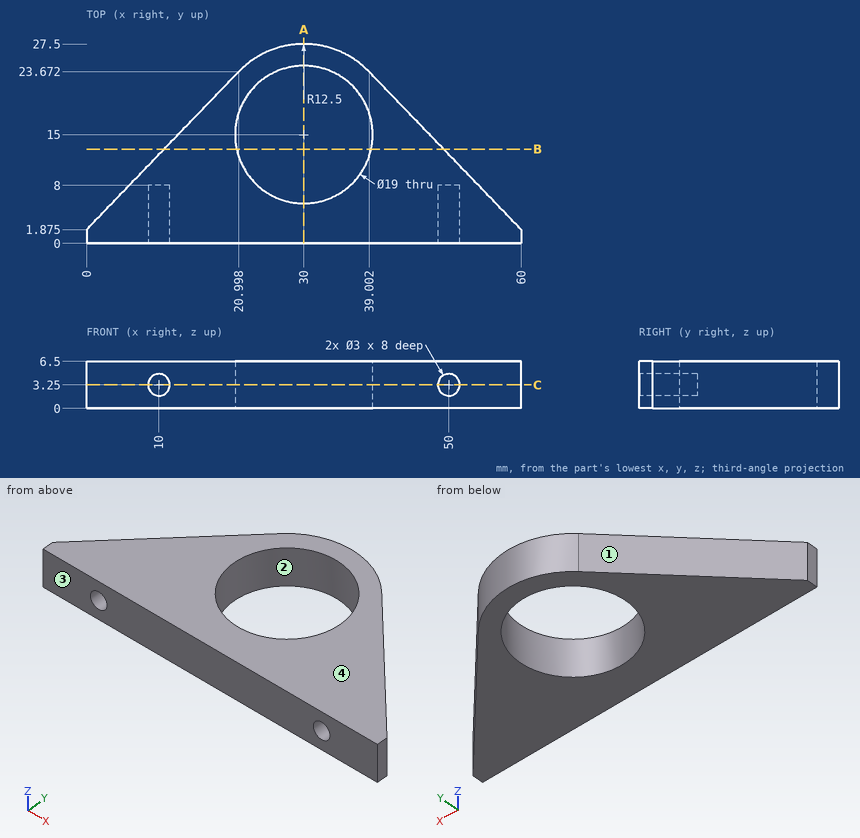
For this review, use the dimensioned drawing (mm, ordinates from the lowest corner) and the shaded views. Give positions to 0.01 mm unless a question says otherwise; leave off trailing zeros. Loops run counter-clockwise (first coordinate to the right, second up) from the corner with the lowest first, then second, coordinate; pieces in that order, holes last.
Item 1: Take a section at A-A, the plane x = 30. State the section outline as (y, z) points.
Item 2: For line 1 along Z through (x, y) = (10, 2); line 2 along Y through (x, z) = (25, 6) (1 decimal); line 3 along X through (y, z) = (15.5, 0.5) (1 decimal), list the stretches that pass through material, from the lowest coordinate up.
Item 3: Draft analysis for pull direction Y (two halves, no side actions). For the marked faces 1, 2, 3 and 4, state which applies: +Y half, -Y half, draft (parallel to the pull), parting line (faces both ways), or undercut.
Item 4: Take a section at C-C, the plane z = 3.25. State the section outline as (x, y) points (1 decimal).
Item 5: Insertion check: pin 1 (1.5 mm diameter, centred on y = 7.5, z = 1.5, fed in from +X) (1 decimal); pin 2 (1.5 mm diameter, centred on y = 5.5, z = 5.5, fed in from +X); pin 3 (0.9 mm diameter, centred on x = 9.5, z = 4, fed in from -Y). Each pin has a flat end and moves straight along its axis. Give the tip position at first contact, or say it passes through.
Item 6: Take a section at B-B, the plane y = 13. State the section outline as (x, z) points, and give its area (3 significant figures).
Calculated:
1. outline: (0, 0) - (5.5, 0) - (5.5, 6.5) - (0, 6.5) - close; (24.5, 0) - (27.5, 0) - (27.5, 6.5) - (24.5, 6.5) - close
2. line 1: z = 0 to 1.75, 4.75 to 6.5
2. line 2: y = 0 to 6.9, 23.1 to 26.5
2. line 3: x = 13.1 to 20.5, 39.5 to 46.9
3. face 1: +Y half
3. face 2: undercut
3. face 3: -Y half
3. face 4: draft
4. outline: (0, 0) - (8.5, 0) - (8.5, 8) - (11.5, 8) - (11.5, 0) - (48.5, 0) - (48.5, 8) - (51.5, 8) - (51.5, 0) - (60, 0) - (60, 1.9) - (39, 23.7) arc R12.5 ccw to (21, 23.7) - (0, 1.9) - close; hole circle Ø19 at (30, 15)
5. pin 1: stops at x = 55.3
5. pin 2: stops at x = 57.23
5. pin 3: stops at y = 8
6. outline: (10.72, 0) - (20.71, 0) - (20.71, 6.5) - (10.72, 6.5) - close; (39.29, 0) - (49.28, 0) - (49.28, 6.5) - (39.29, 6.5) - close
6. area: 130 mm2
